from build123d import *

# Parameters (mm, degrees)
F0_W     = 76.2
F0_H     = 152.4
F1_DEPTH = 19.05
F3_D     = 5.1054
F3_DEPTH = 25.4
F3_TIP   = 1.5338169022
F4_D     = 5.1054
F4_DEPTH = 25.4
F4_TIP   = 1.5338169022
F6_D     = 5.1054
F6_DEPTH = 25.4
F6_TIP   = 1.5338169022
F7_SIZE  = 12.7


with BuildPart() as f1:
    # F0 (on Front) → F1 (new body)
    with BuildSketch(Plane.XZ):
        with Locations((-38.1, 76.2)):
            Rectangle(F0_W, F0_H)
    extrude(amount=F1_DEPTH)

    # F3
    with Locations(Plane(origin=(0, 0, 0), x_dir=(1, 0, 0), z_dir=(0, 0, -1))):
        with Locations((-50.8, 9.525)):
            Hole(F3_D / 2, depth=F3_DEPTH)
            with Locations((0, 0, -(F3_DEPTH + F3_TIP / 2))):  # 118° drill point
                Cone(0, F3_D / 2, F3_TIP, mode=Mode.SUBTRACT)

    # F4
    with Locations(Plane(origin=(0, 0, 0), x_dir=(1, 0, 0), z_dir=(0, 0, -1))):
        with Locations((-25.4, 9.525)):
            Hole(F4_D / 2, depth=F4_DEPTH)
            with Locations((0, 0, -(F4_DEPTH + F4_TIP / 2))):  # 118° drill point
                Cone(0, F4_D / 2, F4_TIP, mode=Mode.SUBTRACT)

    # F6
    with Locations(Plane.XY.offset(152.4)):
        with Locations((-57.15, -9.525), (-6.35, -9.525)):
            Hole(F6_D / 2, depth=F6_DEPTH)
            with Locations((0, 0, -(F6_DEPTH + F6_TIP / 2))):  # 118° drill point
                Cone(0, F6_D / 2, F6_TIP, mode=Mode.SUBTRACT)

    # F7
    f7_edges = [f1.edges().sort_by_distance(p)[0] for p in [
        (-76.2, -9.525, 152.4),
    ]]
    chamfer(f7_edges, length=F7_SIZE)


solid = f1.part
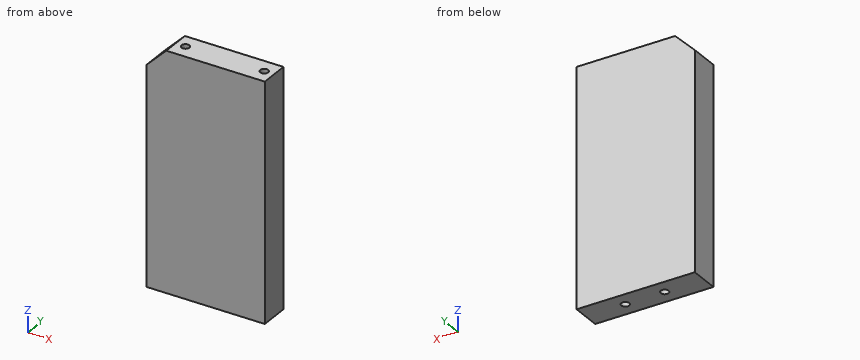
CAD build for the part. Positions are in the model's coordinates, mm. Coordinates: 2 decimals unless noted, no trailing zeros. Order: outer loops, then holes, each group sorted by start corner. A loop starts at its lowest first (then second) coordinate and runs counter-clockwise, first axis right, second up.
Item 1: Drill centre lines: L1, parallel to Y at x = -6.35, z = 145.5; L2, parallel to X at y = -10.75, z = 21; L3, parallel to X at y = -8.25, z = 134. Where is each one in solid material? Low to high.
Check sheet entries:
L1: y = -19.05 to -12.08, -6.97 to 0
L2: x = -76.2 to -53.04, -48.56 to -27.64, -23.16 to 0
L3: x = -76.2 to -59.36, -54.94 to -8.56, -4.14 to 0
Item 2: Pin check, flat tips, straight feed: pin 1 Ø4.5 at (x, y) = (-6.35, -9.525) entering from +Z; pin 2 Ø3 at (x, y) = (-25.4, -9.525) entering from -Z. Stop position of each tip, or through.
Check sheet entries:
pin 1: stops at z = 126.82
pin 2: stops at z = 26.03
Item 3: Band-saw the part on A-A on x = -66. List the corners of the cut face in (y, z).
Check sheet entries:
outline: (-19.05, 0) - (0, 0) - (0, 149.9) - (-19.05, 149.9) - close
